The model under review builds one solid part; all positions refer to its coordinate system, in mm. A direction names the side the tool comes from. Coordinates: 2 decimals unless noted, no trailing zeros. Loops run counter-clockwise (first coordinate to the right, second up) from the corner with the lowest first, then second, coordinate; pieces in that order, holes last. Notation, with made-up numbers: (12.25, 7) - (41.25, 7) arc R30 ccw to (41.25, 31) - close; hole circle Ø7 at (71, -39.5). An arc over 180 degrees is marked (long way). Use a Markdown table: item, result. Add a question column.
1) Clearance check with flat-ended pins moving along their axes: pin 1 (3 mm diameter, centred on x = 4.5, z = -3.5, fed in from +Y); pin 2 (1 mm diameter, centred on x = 4.5, y = -1, fed in from +Z); pin 3 (1.5 mm diameter, centred on x = 6.5, z = -6, fed in from -Y). State where each tip first meets the part, or that it passes through.
2) Add section C-C, the plane x = 1.75. Give the boundary of the cut face in (y, z), and give its area (3 significant figures).
3) Add section D-D, the plane z = -2.75. Give the boundary of the cut face in (x, y).
4) For faces 1 (the flat face through (3, 0, -2)), 2 (the cylindrical face through (4.541, 0.394, -5.467)), 3 (the flat face through (2.83, 2.8, -4.11)), 4 (the flat face through (3.9, 1.5, -7.7)), list the 3-axis set-ups (+Z, -Z, +X, -X, +Y, -Y) from which the entire face can be reached by the end or side of a thin tool; tool diameter is ignored.
5) To check wall thickness, follow L1, parallel to Y at x = 5, z = -4.75; L2, parallel to Z at x = 4.75, y = -1.3; L3, parallel to Y at x = 5.5, z = -5.75. State the ranges of each line that lie inside material, in increasing order. Write a range as [from, to].
6) Add section A-A, the plane y = 0.35. Give the boundary of the cut face in (x, z), and give its area (3 significant figures).
7) Add section B-B, the plane z = -5. Give the boundary of the cut face in (x, y), and give its area (3 significant figures).
8) The part is to be moulded in two halves that separate along Z. For faces 5 (the flat face through (3.9, 1.5, -0.3)), 6 (the flat face through (5.164, 2.803, -4.17)), 7 (the flat face through (0.3, 1.5, -4.1)), say which applies: pulls with the +Z half, pulls with the -Z half, needs draft (parallel to the pull), parting line crosses it, or undercut.
```python
from build123d import *

# Parameters (mm, degrees)
SKETCH1_W               = 8
SKETCH1_H               = 8
BOSS_EXTRUDE1_DEPTH     = 3
CUT_EXTRUDE1_DEPTH      = 12.704699911
CUT_EXTRUDE1_DEPTH_BACK = 12.704699911
CUT_EXTRUDE2_DEPTH      = 11
SKETCH4_R               = 1.8
CUT_EXTRUDE3_DEPTH      = 0.8
SKETCH5_W               = 8
SKETCH5_H               = 1
BOSS_EXTRUDE2_DEPTH     = 2
FILLET1_R               = 4
CUT_EXTRUDE4_DEPTH      = 0.4


with BuildPart() as part:
    # Sketch1 → Boss-Extrude1 (new body)
    with BuildSketch(Plane(origin=(0, 0, 0), x_dir=(1, 0, 0), z_dir=(0, 1, 0))):
        with Locations((4, 4)):
            Rectangle(SKETCH1_W, SKETCH1_H)
    extrude(amount=BOSS_EXTRUDE1_DEPTH)

    # Sketch2 → Cut-Extrude1 (cut, two sides: drawn at the far end of the back side and taken through both)
    with BuildSketch(Plane.XY.offset(-CUT_EXTRUDE1_DEPTH_BACK)):
        Polygon((0, 0), (0.6, 3), (0, 3), align=None)
        Polygon((8, 0), (7.4, 3), (8, 3), align=None)
    extrude(amount=CUT_EXTRUDE1_DEPTH + CUT_EXTRUDE1_DEPTH_BACK, mode=Mode.SUBTRACT)

    # Sketch3 → Cut-Extrude2 (cut)
    with BuildSketch(Plane(origin=(0, 0, 0), x_dir=(0, 0, -1), z_dir=(1, 0, 0))):
        Polygon((0, 0), (0.6, 3), (0, 3), align=None)
        Polygon((8, 3), (7.4, 3), (8, 0), align=None)
    extrude(amount=CUT_EXTRUDE2_DEPTH, mode=Mode.SUBTRACT)

    # Sketch4 → Cut-Extrude3 (cut)
    with BuildSketch(Plane.XZ):
        with Locations(Location((4, -3.75, 0), (0, 0, 270))):
            Circle(SKETCH4_R)
    extrude(amount=-CUT_EXTRUDE3_DEPTH, mode=Mode.SUBTRACT)

    # Sketch5 → Boss-Extrude2 (add)
    with BuildSketch(Plane.XZ):
        with Locations((4, -7.5)):
            Rectangle(SKETCH5_W, SKETCH5_H)
    extrude(amount=BOSS_EXTRUDE2_DEPTH)

    # Fillet1
    # the kernel refuses this fillet: 4 mm, written as the material it takes off along each edge
    with BuildSketch(Plane(origin=(8, -2, -16.660254038), x_dir=(0, 1, 0), z_dir=(0, 0, 1)), Plane(origin=(0, -2, 1.660254038), x_dir=(0, 1, 0), z_dir=(0, 0, -1))) as fillet1_piece_1:
        with BuildLine():
            CenterArc((4, 3.464101615), FILLET1_R, 180, 60)
            Line((0, 3.464101615), (-0.08, 3.464101615))
            Line((-0.08, 3.464101615), (-0.08, 0))
            Line((-0.08, 0), (0, -0.08))
            ThreePointArc((0, -0.08), (1, -0.08), (1.96, -0.069282032))
            Line((1.96, -0.069282032), (2, 0))
        make_face()
    extrude(amount=18.320508076, mode=Mode.SUBTRACT)

    # Sketch6 → Cut-Extrude4 (cut)
    with BuildSketch(Plane(origin=(0, 3, 0), x_dir=(1, 0, 0), z_dir=(0, 1, 0))):
        Polygon((5.933857302, 2.141652068), (5.118152174, 2.141652068), (4.780812431, 3.064728992), (3.24555602, 3.064728992), (2.908216277, 2.141652068), (2.087703456, 2.141652068), (3.599722687, 6.141652068), (4.414626533, 6.141652068), align=None)
        Polygon((4.536421405, 3.731395658), (4.010780379, 5.167293094), (3.486741918, 3.731395658), align=None, mode=Mode.SUBTRACT)
    extrude(amount=-CUT_EXTRUDE4_DEPTH, mode=Mode.SUBTRACT)


solid = part.part
```
From the geometry:
| question | item | result |
|---|---|---|
| 1 | pin 1 | stops at y = 3 |
| 1 | pin 2 | stops at z = -7 |
| 1 | pin 3 | stops at y = 0 |
| 2 | outline | (-1.61, -8) - (0, -8) - (3, -7.4) - (3, -0.6) - (0, 0) - (0, -7) - (-1.61, -7) - close |
| 2 | area | 23.8 mm^2 |
| 3 | outline | (0, 0) - (2.5, 0) - (2.5, 0.8) - (5.5, 0.8) - (5.5, 0) - (8, 0) - (7.4, 3) - (5.7, 3) - (5.7, 2.6) - (4.9, 2.6) - (4.9, 3) - (3.13, 3) - (3.13, 2.6) - (2.32, 2.6) - (2.32, 3) - (0.6, 3) - close |
| 4 | face 1 | +Z, +X, -X, -Y |
| 4 | face 2 | -Y |
| 4 | face 3 | +Y |
| 4 | face 4 | -Z, +X, -X, +Y |
| 5 | L1 | y = [0.8, 3] |
| 5 | L2 | z = [-8, -7] |
| 5 | L3 | y = [0, 3] |
| 6 | outline | (0.07, -7.93) - (7.93, -7.93) - (7.93, -0.07) - (0.07, -0.07) - close; hole circle Ø3.6 at (4, -3.75) |
| 6 | area | 51.6 mm^2 |
| 7 | outline | (0, 0) - (2.7, 0) - (2.7, 0.8) - (5.3, 0.8) - (5.3, 0) - (8, 0) - (7.4, 3) - (4.85, 3) - (4.85, 2.6) - (4.07, 2.6) - (4.07, 3) - (3.95, 3) - (3.95, 2.6) - (3.17, 2.6) - (3.17, 3) - (0.6, 3) - close |
| 7 | area | 19.5 mm^2 |
| 8 | face 5 | pulls with the +Z half |
| 8 | face 6 | undercut |
| 8 | face 7 | needs draft |
